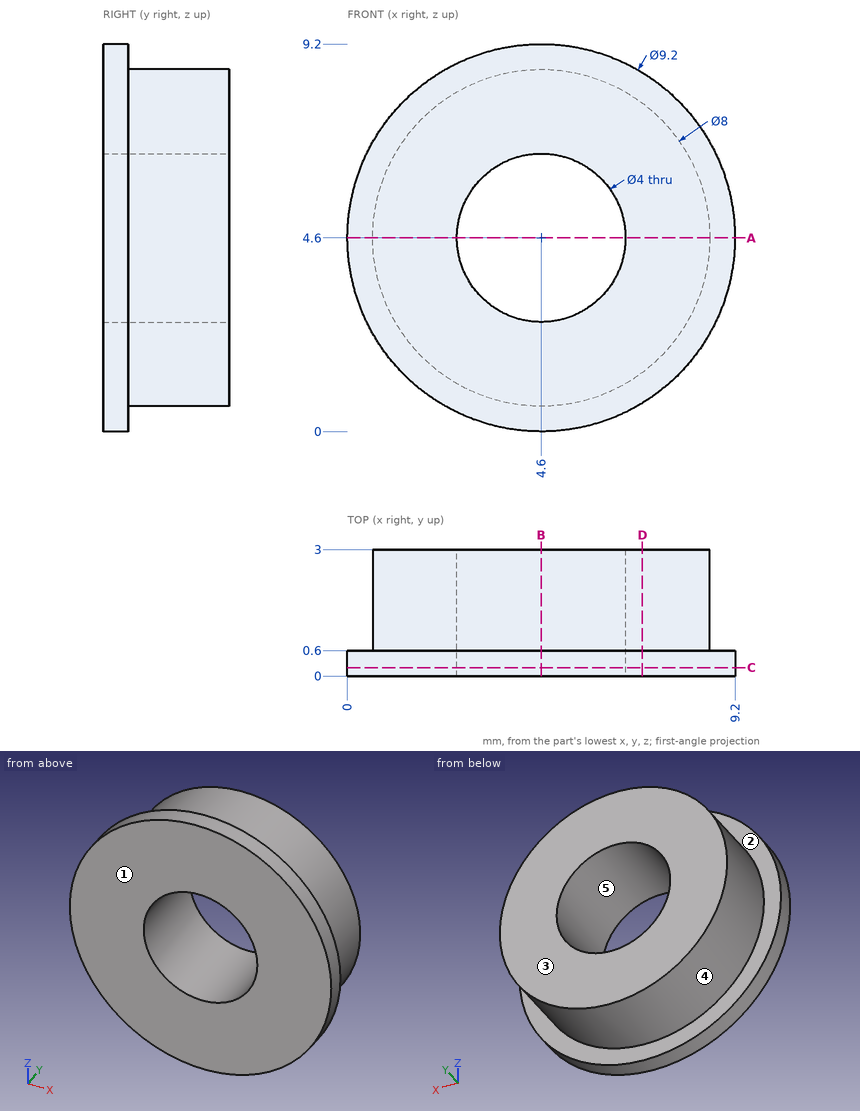
Geometry check sheet. Reference: drawing and pictorial views, mm from the part's lowest x, y, z. A direction names the side the tool comes from. Coordinates: 2 decimals unless noted, no trailing zeros. Write each loop counter-clockwise with the first axis right and the second up, starting at its lowest first coordinate (ties: lowest second). Pieces come first, ordered by that corner, then holes. Notation, with made-up numbers: (-15, 40) -> (-11, 40) arc R33 cw to (-11, 76) -> close; hole circle Ø10 at (59.25, 12.5). An arc over 180 degrees is marked (long way). One line per question, with ' | ' between items.
1. Thickness scan on probe 1 along Z at (x, y) = (4.6, 2.45); probe 2 along Z at (x, y) = (4.5, 0.5). Record the ranges inside material, lowest first. Write a range as from..to.
Answers:
probe 1: z = 0.6..2.6, 6.6..8.6 | probe 2: z = 0..2.6, 6.6..9.2
2. Cross-section at A-A on z = 4.6. Record the cut outline in (x, y), and give its area (3 significant figures).
Answers:
outline: (0, 0) -> (2.6, 0) -> (2.6, 3) -> (0.6, 3) -> (0.6, 0.6) -> (0, 0.6) -> close; (6.6, 0) -> (9.2, 0) -> (9.2, 0.6) -> (8.6, 0.6) -> (8.6, 3) -> (6.6, 3) -> close | area: 12.7 mm²
3. Draft check along Z on the marked faces 3, 4 and 5. Enter one of: +Z half, -Z half, draft (parallel to the pull), parting line (faces both ways), or undercut.
Answers:
face 3: draft | face 4: parting line | face 5: undercut
4. Cross-section at D-D on x = 7. Record the cut outline in (y, z).
Answers:
outline: (0, 0.68) -> (0.6, 0.68) -> (0.6, 1.4) -> (3, 1.4) -> (3, 7.8) -> (0.6, 7.8) -> (0.6, 8.52) -> (0, 8.52) -> close
5. Cross-section at B-B on x = 4.6. Record the cut outline in (y, z).
Answers:
outline: (0, 0) -> (0.6, 0) -> (0.6, 0.6) -> (3, 0.6) -> (3, 2.6) -> (0, 2.6) -> close; (0, 6.6) -> (3, 6.6) -> (3, 8.6) -> (0.6, 8.6) -> (0.6, 9.2) -> (0, 9.2) -> close
6. Depth check by flat-ended pin: pin 1 Ø3.5 at (x, z) = (4.6, 4.6) entering from -Y. Enter the tip coordinate at first touch or a pass-through.
Answers:
pin 1: passes through
7. Set-up check for the marked faces 1 and 2: record each of +Z, -Z, +X, -X, +Y, -Y from which the full face is reachable in a straight line by a thin tool's end or side.
Answers:
face 1: +Z, -Z, +X, -X, -Y | face 2: +Y
8. Cross-section at C-C on y = 0.2. Record the cut outline in (x, z).
Answers:
outline: circle Ø9.2 at (4.6, 4.6); hole circle Ø4 at (4.6, 4.6)
